CAD build for the part. Positions are in the model's coordinates, mm. A direction names the side the tool comes from. Coordinates: 2 decimals unless noted, no trailing zeros. Loops run counter-clockwise (first coordinate to the right, second up) from the corner with the lowest first, then second, coordinate; pieces in that order, holes last. Notation, with made-up numbers: (82.5, 81.5) -> (132.5, 81.5) arc R25 cw to (132.5, 102.5) -> close; hole circle Ø3 at (75.25, 12.5). An arc over 180 degrees is marked (long way). Write each question's results on one line, items separated by ' | '.
Autodesk Inventor part; units mm, degrees
ref_plane "YZ Plane" through (0, 0, 0) normal (1, 0, 0) x (0, 1, 0)
ref_plane "XZ Plane" through (0, 0, 0) normal (0, 1, 0) x (-1, 0, 0)
ref_plane "XY Plane" through (0, 0, 0) normal (0, 0, 1) x (1, 0, 0)
sketch "スケッチ1" plane through (0, 0, 0) normal (0, 0, 1) x (1, 0, 0)
  circle A0 centre (-20, 0) radius 1.6
  circle A1 centre (20, 0) radius 1.6
  circle A2 centre (0, 0) radius 1.6
  circle A3 centre (-87.5, 27.5) radius 1.6
  circle A4 centre (87.5, 27.5) radius 1.6
  arc A5 (-87.5, 32.5) -> (-89.5442, 22.937) centre (-87.5, 27.5) ccw
  arc A6 (89.5442, 22.937) -> (87.5, 32.5) centre (87.5, 27.5) ccw
  arc A7 (20, -7.5) -> (23.0663, -6.8445) centre (20, 0) ccw
  arc A8 (-23.0663, -6.8445) -> (-20, -7.5) centre (-20, 0) ccw
  line L0 (-89.5442, 22.937) -> (-23.0663, -6.8445)
  line L1 (-87.5, 32.5) -> (87.5, 32.5)
  line L2 (89.5442, 22.937) -> (23.0663, -6.8445)
  line L3 (20, -7.5) -> (-20, -7.5)
  dimension "d0" = 3.2
  dimension "d1" = 3.2
  dimension "d2" = 3.2
  dimension "d3" = 20
  dimension "d4" = 20
  dimension "d5" = 3.2
  dimension "d6" = 3.2
  dimension "d14" = 175
  dimension "d15" = 87.5
  dimension "d17" = 5
  dimension "d18" = 5
  dimension "d19" = 7.5
  dimension "d20" = 7.5
  dimension "d23" = 27.5
extrude "押し出し1" add sketch "スケッチ1" along normal blind 3
sketch "スケッチ2" plane through (0, 0, 3) normal (0, 0, 1) x (1, 0, 0)
  circle A0 centre (-87.5, 27.5) radius 1.6
  arc A1 (-82.937, 25.4558) -> (-82.601, 28.5) centre (-87.5, 27.5) ccw
  circle A2 centre (87.5, 27.5) radius 1.6
  arc A3 (82.601, 28.5) -> (82.937, 25.4558) centre (87.5, 27.5) ccw
  line L0 (-82.601, 28.5) -> (82.601, 28.5)
  line L1 (87.5, 32.5) -> (-87.5, 32.5)
  line L2 (-18.3968, 7.5) -> (18.3968, 7.5)
  line L3 (18.3968, 7.5) -> (82.937, 25.4558)
  line L4 (-18.3968, 7.5) -> (-82.937, 25.4558)
  line L5 (-20, -7.5) -> (20, -7.5)
  line L6 (-89.5442, 22.937) -> (-23.0663, -6.8445)
  line L7 (23.0663, -6.8445) -> (89.5442, 22.937)
  point P0 (0, 0)
  dimension "d24" = 5
  dimension "d25" = 5
  dimension "d26" = 4
  dimension "d27" = 15
  dimension "d28" = 15
  dimension "d29" = 15
  dimension "d30" = 5
  dimension "d31" = 5
extrude "押し出し2" cut sketch "スケッチ2" against normal through all contours A1 L0 A3 L3 L2 L4
fillet "フィレット1" radius 2 6 edges at (-82.601, 28.5, 1.5) (-82.937, 25.4558, 1.5) (-18.3968, 7.5, 1.5) (18.3968, 7.5, 1.5) (82.601, 28.5, 1.5) (82.937, 25.4558, 1.5)
properties part number "ハンド_上側板" material "アルミニウム 6061"
Q1. Pull direction Y, two halves, no side cores. Call faces 1 (the cylindrical face through (21.59, -7.33, 1.48)), 2 (the cylindrical face through (18.82, -1.08, 1.48)), 3 (the flat face through (-1, 32.5, 1)): +Y half, -Y half, draft (parallel to the pull), parting line (faces both ways), or undercut.
Results are:
face 1: -Y half | face 2: undercut | face 3: +Y half
Q2. Wall check: L1, parallel to Y at x = 0, z = 1.55; L2, parallel to X at y = 28, z = 1.1; L3, parallel to Y at x = -51, z = 2.4. Give the ranges that are in metal, low to high. Write a range as from..to.
Results are:
L1: -7.5..-1.6, 1.6..7.5, 28.5..32.5 | L2: -92.47..-89.02, -85.98..-80.56, 80.56..85.98, 89.02..92.47 | L3: 5.67..16.57, 28.5..32.5
Q3. Drop flat-ended pins along their axis: pin 1 (1 mm diameter, centred on y = 1, z = 2.5, fed in from -X); pin 2 (1.5 mm diameter, centred on y = 13, z = 0.5, fed in from -X). Give the stop position or say it passes through.
Results are:
pin 1: x = -41.69 | pin 2: x = -69.04
Q4. Cut at B-B on y = 0. Write the cut outline in (x, z), and give its area (3 significant figures).
Results are:
outline: (-38.34, 0) -> (-21.6, 0) -> (-21.6, 3) -> (-38.34, 3) -> close; (-18.4, 0) -> (-1.6, 0) -> (-1.6, 3) -> (-18.4, 3) -> close; (1.6, 0) -> (18.4, 0) -> (18.4, 3) -> (1.6, 3) -> close; (21.6, 0) -> (38.34, 0) -> (38.34, 3) -> (21.6, 3) -> close | area: 201 mm^2
Q5. Cut at A-A on x = 0. Write the cut outline in (y, z).
Results are:
outline: (-7.5, 0) -> (-1.6, 0) -> (-1.6, 3) -> (-7.5, 3) -> close; (1.6, 0) -> (7.5, 0) -> (7.5, 3) -> (1.6, 3) -> close; (28.5, 0) -> (32.5, 0) -> (32.5, 3) -> (28.5, 3) -> close
Q6. Cut at C-C on x = -60.5. Write the cut outline in (y, z), and give its area (3 significant figures).
Results are:
outline: (9.93, 0) -> (19.21, 0) -> (19.21, 3) -> (9.93, 3) -> close; (28.5, 0) -> (32.5, 0) -> (32.5, 3) -> (28.5, 3) -> close | area: 39.9 mm^2
Q7. Cut at D-D on z = 0.85. Give the number of separate pieces and of enclosed holes in the cut face, and give its area (3 significant figures).
Results are:
separate pieces: 1 | enclosed holes: 6 | area: 2,780 mm^2
Q8. Which spindle directions (+Z, -Z, +X, -X, +Y, -Y) get a long thin tool onto all of the face, cutting with end or side? Do faces 4 (the flat face through (-1, 4, 0)), 5 (the flat face through (0, 7.5, 2)). Say none if no direction does.
Results are:
face 4: -Z, +X, -X, +Y, -Y | face 5: +Z, -Z
